Here's how the part is built. I have some questions about the finished solid (model axes, mm). Coordinates: 2 decimals unless noted, no trailing zeros. Write each loop counter-clockwise with the first axis right and the second up, starting at its lowest first coordinate (ties: lowest second). Pieces come first, ordered by that corner, then holes.
Item 1: Please list where these lines run through material, in increasing order: line 1 (Y direction, x = 50, z = -10.5); line 2 (X direction, y = 13, z = -21.5); line 3 (X direction, y = 9.5, z = -32).
Item 2: I want a section at C-C (x = 50). Please give me the cut outline in (y, z), and give its area (3 significant figures).
Item 3: I want a section at B-B (y = 35). Please give me the cut outline in (x, z), and give its area (3 significant figures).
Item 4: I want a section at A-A (x = 110). Please give me the cut outline in (y, z), and give its area (3 significant figures).
Item 5: If we mould it in two halves opening along X, with no side actions, what happens to faces 1 (the face through (76.05, 57.15, -36.99)), 2 (the face through (105.904, 35.18, -21.266)), 3 (the face through (157.15, 24.65, -36.99))? For each: pulls with the +X half, pulls with the -X half, needs draft (parallel to the pull), parting line crosses it, or undercut.
Item 6: I want a section at D-D (z = -5). Please give me the cut outline in (x, y).
from build123d import *

# Parameters (mm, degrees)
SKETCH1_W                  = 80
SKETCH1_H                  = 40
CNFBOSS_EXTRUDE1_DEPTH     = 60
SKETCH2_R                  = 5
CNFCUT_DEPTH               = 108.703296143
F_8_2_8_2_DIAMETER_HOLE1_D = 8.2
CNFFILLET_R                = 10
CNFFILLET2_R               = 10
CNFCHAMFER_SIZE            = 2


with BuildPart() as part:
    # Sketch1 → cnfBoss-Extrude1 (new body)
    with BuildSketch(Plane(origin=(0, 0, 0), x_dir=(1, 0, 0), z_dir=(0, 1, 0))):
        with Locations((40, 20)):
            Rectangle(SKETCH1_W, SKETCH1_H)
    extrude(amount=CNFBOSS_EXTRUDE1_DEPTH)

    # Sketch2 → cnfCut (cut, through all)
    with BuildSketch(Plane.XY):
        with Locations((12.01333081, 11.907221875)):
            Circle(SKETCH2_R)
    extrude(amount=-CNFCUT_DEPTH, mode=Mode.SUBTRACT)

    # Ø8.2 (8.2) Diameter Hole1 (through all)
    with Locations(Plane.XY):
        with Locations((50, 35)):
            Hole(F_8_2_8_2_DIAMETER_HOLE1_D / 2)

    # cnfMirror: part across plane


with BuildPart() as part_1:
    add(part.part)
    add(part.part.mirror(Plane(origin=(80, 60, 0), x_dir=(0, 0, 1), z_dir=(-1, 0, 0))))

    # cnfFillet
    # the kernel refuses this fillet: 10 mm, written as the material it takes off along each edge
    with BuildSketch(Plane(origin=(160, -25, -40), x_dir=(-1, 0, 0), z_dir=(0, 1, 0))) as cnffillet_piece_1:
        with BuildLine():
            CenterArc((CNFFILLET_R, CNFFILLET_R), CNFFILLET_R, 180, 90)
            Line((0, CNFFILLET_R), (0, 0))
            Line((0, 0), (CNFFILLET_R, 0))
        make_face()
    extrude(amount=110, mode=Mode.SUBTRACT)

    # cnfFillet2
    cnffillet2_edges = [part_1.edges().sort_by_distance(p)[0] for p in [
        (75, 60, -40),
        (160, 60, -15),
        (157.071067812, 60, -37.071067812),
    ]]
    fillet(cnffillet2_edges, radius=CNFFILLET2_R)

    # cnfChamfer
    cnfchamfer_edges = [part_1.edges().sort_by_distance(p)[0] for p in [
        (105.9, 35, 0),
    ]]
    chamfer(cnfchamfer_edges, length=CNFCHAMFER_SIZE)


solid = part_1.part
Answer:
1. line 1: y = 0 to 30.9, 39.1 to 60
1. line 2: x = 0 to 7.13, 16.89 to 143.11, 152.87 to 160
1. line 3: x = 0 to 7.63, 16.4 to 143.6, 152.37 to 159.8
2. outline: (0, -40) - (30.9, -40) - (30.9, 0) - (0, 0) - close; (39.1, -40) - (50, -40) arc R10 ccw to (60, -30) - (60, 0) - (39.1, 0) - close
2. area: 2,050 mm2
3. outline: (0, -40) - (45.9, -40) - (45.9, 0) - (0, 0) - close; (54.1, -40) - (105.9, -40) - (105.9, -2) - (103.9, 0) - (54.1, 0) - close; (114.1, -40) - (150, -40) arc R10 ccw to (160, -30) - (160, 0) - (116.1, 0) - (114.1, -2) - close
3. area: 5,720 mm2
4. outline: (0, -40) - (30.9, -40) - (30.9, -2) - (28.9, 0) - (0, 0) - close; (39.1, -40) - (50, -40) arc R10 ccw to (60, -30) - (60, 0) - (41.1, 0) - (39.1, -2) - close
4. area: 2,050 mm2
5. face 1: needs draft
5. face 2: undercut
5. face 3: pulls with the +X half
6. outline: (0, 0) - (160, 0) - (160, 50) arc R10 ccw to (150, 60) - (0, 60) - close; hole circle Ø10 at (12.01, 11.91); hole circle Ø8.2 at (50, 35); hole circle Ø8.2 at (110, 35); hole circle Ø10 at (147.99, 11.91)
